Autodesk Inventor part; units mm, degrees
ref_plane "YZ Plane" through (0, 0, 0) normal (1, 0, 0) x (0, 1, 0)
ref_plane "XZ Plane" through (0, 0, 0) normal (0, 1, 0) x (-1, 0, 0)
ref_plane "XY Plane" through (0, 0, 0) normal (0, 0, 1) x (1, 0, 0)
sketch "Sketch1" plane through (0, 0, 0) normal (0, 0, 1) x (1, 0, 0)
  arc A0 (-46.3925, 24.0714) -> (-43.8475, 26.6164) centre (-45.0925, 25.3164) ccw
  line L0 (-46.3925, 9.0304) -> (-46.3925, 24.0714)
  line L1 (-46.3925, 9.0304) -> (-44.3931, 9.0304)
  line L2 (-44.3925, 21.1036) -> (-44.3931, 9.0304)
  arc A1 (-44.3925, 21.1036) -> (-40.8797, 24.6164) centre (-43.8925, 24.1164) ccw
  line L3 (40.9925, 24.6164) -> (-40.8797, 24.6164)
  line L4 (40.9925, 16.6164) -> (40.9925, 24.6164)
  line L5 (44.3925, 16.6164) -> (40.9925, 16.6164)
  line L6 (44.3925, 2.4144) -> (44.3925, 16.6164)
  line L7 (44.3925, 2.4144) -> (46.3925, 2.4144)
  line L8 (46.3925, 24.0714) -> (46.3925, 2.4144)
  arc A2 (43.8475, 26.6164) -> (46.3925, 24.0714) centre (45.0925, 25.3164) ccw
  line L9 (-43.8475, 26.6164) -> (43.8475, 26.6164)
  arc A3 (-43.8475, -26.6164) -> (-46.3925, -24.0714) centre (-45.0925, -25.3164) ccw
  line L10 (43.8475, -26.6164) -> (-43.8475, -26.6164)
  arc A4 (46.3925, -24.0714) -> (43.8475, -26.6164) centre (45.0925, -25.3164) ccw
  line L11 (46.3925, -21.5856) -> (46.3925, -24.0714)
  line L12 (46.3925, -21.5856) -> (44.3925, -21.5856)
  line L13 (44.3925, -19.6418) -> (44.3925, -21.5856)
  line L14 (40.3925, -19.6418) -> (44.3925, -19.6418)
  line L15 (40.3925, -24.6418) -> (40.3925, -19.6418)
  line L16 (-40.8818, -24.6418) -> (40.3925, -24.6418)
  arc A5 (-40.8818, -24.6418) -> (-42.6446, -21.3551) centre (-43.8945, -24.1416) ccw
  line L17 (-46.3925, -21.3551) -> (-42.6446, -21.3551)
  line L18 (-46.3925, -24.0714) -> (-46.3925, -21.3551)
  line L19 (-46.3925, -21.7457) -> (-46.3925, -24.0714)
  arc A6 (-46.3925, -21.7457) -> (-41.5218, -26.6164) centre (-45.0925, -25.3164) ccw
  line L20 (-43.8475, -26.6164) -> (-41.5218, -26.6164)
  arc A7 (-46.3925, -24.0714) -> (-43.8475, -26.6164) centre (-45.0925, -25.3164) ccw
  line L21 (41.5218, -26.6164) -> (43.8475, -26.6164)
  arc A8 (41.5218, -26.6164) -> (46.3925, -21.7457) centre (45.0925, -25.3164) ccw
  line L22 (46.3925, -24.0714) -> (46.3925, -21.7457)
  arc A9 (43.8475, -26.6164) -> (46.3925, -24.0714) centre (45.0925, -25.3164) ccw
  line L23 (46.3925, 21.7457) -> (46.3925, 24.0714)
  arc A10 (46.3925, 21.7457) -> (41.5218, 26.6164) centre (45.0925, 25.3164) ccw
  line L24 (43.8475, 26.6164) -> (41.5218, 26.6164)
  arc A11 (46.3925, 24.0714) -> (43.8475, 26.6164) centre (45.0925, 25.3164) ccw
  line L25 (-41.5218, 26.6164) -> (-43.8475, 26.6164)
  arc A12 (-41.5218, 26.6164) -> (-46.3925, 21.7457) centre (-45.0925, 25.3164) ccw
  line L26 (-46.3925, 24.0714) -> (-46.3925, 21.7457)
  arc A13 (-43.8475, 26.6164) -> (-46.3925, 24.0714) centre (-45.0925, 25.3164) ccw
  line L27 (44.3925, 2.4144) -> (0, 2.4144)
  line L28 (0, 2.4144) -> (0, 24.6164)
  line L29 (44.3925, -21.5856) -> (0, -21.5856)
  line L30 (-44.3937, -2.9696) -> (-46.3925, -2.9696)
  line L31 (-46.3925, -11.5551) -> (-46.3925, -2.9696)
  line L32 (-44.3941, -11.5551) -> (-46.3925, -11.5551)
  line L33 (-44.3937, -2.9696) -> (-44.3941, -11.5551)
  line L34 (-46.3925, -21.7457) -> (-46.3925, -11.5551)
  line L35 (-46.3925, -2.9696) -> (-46.3925, 9.0304)
  line L36 (0, -11.3836) -> (-27, -11.3836)
  line L37 (-27, -11.3836) -> (-27, 15.6164)
  line L38 (-27, 15.6164) -> (0, 15.6164)
  line L39 (0, 15.6164) -> (0, -11.3836)
  line L40 (0, -11.3836) -> (0, -21.5856)
  point P0 (0, 0)
  point P1 (40.3925, -21.5856)
  point P2 (0, 15.6164)
extrude "Extrusion1" add sketch "Sketch1" along normal blind 3 contours A0 L9 A2 L8 L7 L6 L5 L4 L3 A1 L2 L1 L0 | L0 A12 L9 A13 | L1 L2 A1 L3 L28 L38 L37 L36 L40 L29 L15 L16 A5 L17 L34 L32 L33 L30 L35 | A10 L8 A11 L9 | L17 A5 L16 L15 L29 L12 L11 A4 L10 A3 L18 | L27 L28 L3 L4 L5 L6 | L18 A7 L10 A6 | L10 A9 L11 A8 | L15 L14 L13 L29
sketch "Sketch2" plane through (44.3925, -21.5856, 0) normal (1, 0, 0) x (0, 0, -1)
  line L0 (0, 0) -> (-8, 8)
  line L1 (-8, 16) -> (0, 24)
  line L2 (-8, 8) -> (-8, 16)
  line L3 (-0.0707, -0.0707) -> (-8.1, 7.9586)
  line L4 (-8.1, 7.9586) -> (-8.1, 16.0414)
  line L5 (-8.1, 16.0414) -> (-0.0707, 24.0707)
  line L6 (0, 0) -> (-3, 0)
  line L7 (0, 24) -> (-3, 24)
  line L8 (-3, 0) -> (-10.1, 7.1)
  line L9 (-10.1, 7.1) -> (-10.1, 16.9)
  line L10 (-10.1, 16.9) -> (-3, 24)
  point P0 (0, 21.5856)
  point P1 (-0.1414, 24)
  point P2 (-0.1414, 0)
  dimension "d5" = 0.1
  dimension "d6" = 2
extrude "Extrusion2" add sketch "Sketch2" along normal blind 2 and the other way blind 71.5 contours L6 L8 L9 L10 L7 L5 L4 L3
sketch "Sketch3" plane through (0, 0, 3) normal (0, 0, 1) x (1, 0, 0)
  line L0 (0, 15.6164) -> (0, 2.4144)
  line L1 (-27.1075, -21.5856) -> (-27.1075, -14.4856)
  line L2 (0, 15.6164) -> (-27.1075, 15.6164)
  line L3 (-27.1075, 15.6164) -> (-27.1075, -14.4856)
  line L4 (-27.1075, -14.4856) -> (0, -14.4856)
  line L5 (0, -14.4856) -> (0, 15.6164)
  point P0 (0, 0)
  point P1 (0, 2.4144)
extrude "Extrusion3" cut sketch "Sketch3" along normal blind 10 and the other way blind 3.25
sketch "Sketch4" plane through (0, 2.4144, 0) normal (-1, 0, 0) x (0, 0, 1)
  line L0 (10.1, -16.9) -> (7.2414, -16.9)
  line L1 (8.1, -16.0414) -> (8.1, -7.9586)
  line L2 (8.1, -15.8474) -> (8.1, -16.9)
  line L3 (8.1, -16.9) -> (10.1, -16.9)
  line L4 (10.1, -16.9) -> (10.1, 13.202)
  line L5 (10.1, 13.202) -> (8.1, 13.202)
  line L6 (8.1, 13.202) -> (8.1, -16.9)
  line L7 (10.1, 13.202) -> (2.1168, 21.1852)
  line L8 (10.1, 13.202) -> (21.3899, 13.202) construction
  line L9 (3, 13.202) -> (3, 0)
  line L10 (3, 0) -> (3, 19.3313)
  line L11 (3, 19.3313) -> (3, 24.202)
  line L12 (3, 24.202) -> (3, 19.3313)
  line L13 (3, 19.3313) -> (3, -5.384)
  line L14 (3, -5.384) -> (3, -13.9695)
  line L15 (3, -13.9695) -> (3, -24.1601)
  line L16 (3, -24.1601) -> (3, -29.0308)
  line L17 (3, -29.0308) -> (3, -24.1601)
  line L18 (3, -24.1601) -> (3, -24)
  line L19 (3, -24) -> (3, -21.1414)
  line L20 (3, -21.1414) -> (3, -16.9)
  line L21 (3, -16.9) -> (3, 13.202)
  line L22 (3, 24.702) -> (3, 21.102)
  line L23 (3, -25.9308) -> (3, -29.5308)
  line L24 (3, -25.9308) -> (3, -29.5308)
  line L25 (3, 24.702) -> (3, 21.102)
  line L26 (8.1, 13.202) -> (3, 18.302)
  point P0 (0, -2.4144)
  point P1 (10.1, -7.1)
  point P2 (8.1, -7.9586)
  point P3 (3, 20.302)
  point P4 (3, 18.302)
  dimension "d15" = 135
extrude "Extrusion4" add sketch "Sketch4" along normal up to surface (27.1075 mm away)
sketch "Sketch5" plane through (0, 2.4144, 0) normal (1, 0, 0) x (0, 0, -1)
  line L0 (-10.1, -7.1) -> (-10.1, 13.202)
  line L1 (-8.1, -5.1) -> (-10.1, -7.1)
  line L2 (-8.1, 13.202) -> (-8.1, -5.1)
  line L3 (-3, 18.302) -> (-8.1, 13.202)
  line L4 (-3, 20.302) -> (-3, 18.302)
  line L5 (-10.1, 13.202) -> (-3, 20.302)
  line L6 (-10.1, -7.1) -> (-10.1, 13.202)
  line L7 (-3, 18.302) -> (-3, 0)
  line L8 (-3, 0) -> (-8.1, -5.1)
  point P0 (0, -2.4144)
  point P1 (-10.1, 13.202)
extrude "Extrusion5" add sketch "Sketch5" along normal blind 2
sketch "Sketch6" plane through (-27.1075, -21.5856, 0) normal (-1, 0, 0) x (0, 0, 1)
  line L0 (8.1, 7.1) -> (7.2414, 7.1)
  line L1 (7.2414, 7.1) -> (3, 2.8586)
  line L2 (3, 0) -> (3, 2.8586)
  line L3 (3, 0) -> (10.1, 7.1)
  line L4 (10.1, 37.202) -> (10.1, 7.1)
  line L5 (3, 44.302) -> (10.1, 37.202)
  line L6 (3, 42.302) -> (3, 44.302)
  line L7 (8.1, 37.202) -> (3, 42.302)
  line L8 (8.1, 7.1) -> (8.1, 37.202)
  line L9 (3, 0) -> (14.0396, 0)
  line L10 (14.0396, 0) -> (14.0396, 45.0941)
  line L11 (14.0396, 45.0941) -> (3, 45.0941)
  line L12 (3, 45.0941) -> (3, 0)
  point P0 (0, 21.5856)
  point P1 (3, 2.8586)
extrude "Extrusion6" add sketch "Sketch6" along normal blind 2 contours L8 L7 L6 L5 L4 L3 L2 L1 L0 | L0 L1 L12 L7 L8
sketch "Sketch7" plane through (0, -21.5856, 0) normal (1, 0, 0) x (0, 0, -1)
  line L0 (0, 7.1) -> (-3, 7.1)
  line L1 (-3, 2.8586) -> (-3, 7.1)
  line L2 (-3, 2.8586) -> (-0.1414, 0)
  line L3 (0, 0) -> (-0.1414, 0)
  line L4 (0, 0) -> (0, 7.1)
  point P0 (0, 21.5856)
extrude "Extrusion7" cut sketch "Sketch7" against normal up to surface (27.1075 mm away)
sketch "Sketch8" plane through (0, 0, 3) normal (0, 0, 1) x (1, 0, 0)
  line L0 (35.1595, -0.5396) -> (31.9595, -0.5396)
  line L1 (31.9595, -0.5396) -> (31.9595, 14.6261)
  line L2 (31.9595, 14.6261) -> (35.1595, 14.6261)
  line L3 (35.1595, 14.6261) -> (35.1595, -0.5396)
  line L4 (34.1345, -0.0368) -> (34.1345, -0.9368)
  line L5 (32.9845, -0.0368) -> (32.9845, -0.9368)
  line L6 (32.9845, -0.7101) -> (34.1345, -0.7101)
  line L7 (33.5595, -0.7101) -> (33.5595, 14.6138)
  point P0 (0, 0)
  dimension "d24" = 3.2
  dimension "d25" = 1.6
extrude "Extrusion8" cut sketch "Sketch8" along normal blind 10 and the other way blind 5 contours L0 L1 L2 L3
sketch "Sketch9" plane through (-46.3925, -2.9696, 0) normal (-1, 0, 0) x (0, 0, 1)
  line L0 (-6.415, 12) -> (0, 12)
  line L1 (3, 0) -> (-6.415, 0)
  line L2 (-6.415, 11.8) -> (0, 11.8)
  line L3 (3, 0.2) -> (-6.415, 0.2)
  line L4 (0, 5.384) -> (0, 24.7153)
  arc A0 (0, 9.8) -> (-2, 11.8) centre (-2, 9.8) ccw
  line L5 (0, 24.7153) -> (0, 0)
  arc A1 (-1.8751, 0.2) -> (0, 2.0751) centre (-1.8751, 2.0751) ccw
  point P0 (0, 2.9696)
  dimension "d30" = 0.2
  dimension "d31" = 0.2
  dimension "d32" = 2
properties part number "Top_case"
For this review, take the finished solid that the model builds, in its own axes (mm). A direction names the side the tool comes from. Coordinates: 2 decimals unless noted, no trailing zeros. Order: outer loops, then holes, each group sorted by start corner. A loop starts at its lowest first (then second) coordinate and runs counter-clockwise, first axis right, second up. Notation, with made-up numbers: (6, 72) -> (13, 72) arc R18 ccw to (13, 80) -> close; hole circle Ø10 at (23, -22.5). An arc over 180 degrees is marked (long way). Return JSON: item names as keys, results as strings.
1. Machinability: for faces 5 (the flat face through (46.392, 1.7, 3.5)), 6 (the flat face through (-14, 18, 3)), 7 (the flat face through (40.392, -20, 1)), 8 (the flat face through (31.96, 7, 2)), which of the approach directions +Z, -Z, +X, -X, +Y, -Y give a long, thin tool a straight path to every point of the face, cutting with its end or side? Answer none if there is none.
Answer block:
{"face 5": "+Z, -Z, +X", "face 6": "none", "face 7": "-Z", "face 8": "+Z, -Z"}
2. We need section B-B on x = 34. Write out the cut boundary in (y, z).
Answer block:
{"outline": "(-26.62, 0) -> (-21.59, 0) -> (-21.59, 0.14) -> (-13.63, 8.1) -> (-5.54, 8.1) -> (-0.54, 3.1) -> (-0.54, 5.95) -> (-4.69, 10.1) -> (-14.49, 10.1) -> (-21.59, 3) -> (-26.62, 3) -> close; (14.63, 0) -> (26.62, 0) -> (26.62, 3) -> (14.63, 3) -> close"}
3. For pin 1 Ø0.9 at (x, z) = (11, 2) entering from -Y; pin 2 Ø1 at (y, z) = (18, 3) entering from -X; pin 3 Ø3.5 at (y, z) = (10, 5) entering from +X, all flat-tipped, find the tip position at first contact; note any pin that passes through.
Answer block:
{"pin 1": "y = -26.62", "pin 2": "x = -46.39", "pin 3": "x = 2"}
4. We need section C-C on x = 14. Write out the cut boundary in (y, z), and give its area (3 significant figures).
Answer block:
{"outline": "(-26.62, 0) -> (-21.59, 0) -> (-21.59, 0.14) -> (-13.63, 8.1) -> (-5.54, 8.1) -> (2.41, 0.14) -> (2.41, 0) -> (26.62, 0) -> (26.62, 3) -> (2.41, 3) -> (-4.69, 10.1) -> (-14.49, 10.1) -> (-21.59, 3) -> (-26.62, 3) -> close", "area": "149 mm²"}
5. We need section A-A on y = 11. Write out the cut boundary in (x, z), and give its area (3 significant figures).
Answer block:
{"outline": "(-46.39, 0) -> (-27.11, 0) -> (-27.11, 8.1) -> (0, 8.1) -> (0, 0) -> (31.96, 0) -> (31.96, 3) -> (2, 3) -> (2, 10.1) -> (-29.11, 10.1) -> (-29.11, 3) -> (-46.39, 3) -> close; (35.16, 0) -> (46.39, 0) -> (46.39, 3) -> (35.16, 3) -> close", "area": "270 mm²"}
6. The part is to be moulded in two halves that separate along Z. For faces 1 (the flat face through (1, -6, 8.1)), 2 (the flat face through (0, -3, 10.1)), 3 (the flat face through (-14, 15.616, 1)), 4 (the flat face through (-13.364, 18.131, 5.586)), say which applies: +Z half, -Z half, draft (parallel to the pull), parting line (faces both ways), or undercut.
Answer block:
{"face 1": "-Z half", "face 2": "+Z half", "face 3": "draft", "face 4": "undercut"}
7. For line 1 (X direction, y = 1.5, z = 2.5); line 2 (X direction, y = 1.5, z = 5.5); line 3 (X direction, y = -25, z = 2), list the stretches that pass through material, from the lowest coordinate up. Write a range as from..to.
Answer block:
{"line 1": "-46.39..-27.11, 0..31.96, 35.16..46.39", "line 2": "-29.11..-27.11, 0..2", "line 3": "-48.88..-46.86, -43.32..43.32, 46.86..48.88"}
8. We need section D-D on y = 25. Write out the cut boundary in (x, z), and give its area (3 significant figures).
Answer block:
{"outline": "(-48.88, 0) -> (-46.86, 0) -> (-46.86, 3) -> (-48.88, 3) -> close; (-43.32, 0) -> (43.32, 0) -> (43.32, 3) -> (-43.32, 3) -> close; (46.86, 0) -> (48.88, 0) -> (48.88, 3) -> (46.86, 3) -> close", "area": "272 mm²"}
